from build123d import *

# Parameters (mm, degrees)
F0_W     = 127
F0_H     = 127
F1_DEPTH = 2.54
F2_W     = 127
F2_H     = 127
F2_W_2   = 121.92
F2_H_2   = 121.92
F3_DEPTH = 7.62
F4_W     = 5.08
F4_H     = 6.35
F4_W_2   = 7.62
F5_DEPTH = 15.24
F6_R     = 1.27
F6_W     = 5.08
F6_H     = 2.54
F7_DEPTH = 6.35


# Not quite as in the source:
# - a pattern or mirror of a feature is missing from the dataset's text; its kind, count and spacing are read off the source's solid


with BuildPart() as f1:
    # F0 (on Top) → F1 (new body)
    with BuildSketch(Plane.XY):
        Rectangle(F0_W, F0_H)
    extrude(amount=F1_DEPTH)

    # F2 (on face) → F3 (join)
    with BuildSketch(Plane.XY.offset(2.54)):
        Rectangle(F2_W, F2_H)
        Rectangle(F2_W_2, F2_H_2, mode=Mode.SUBTRACT)
    extrude(amount=F3_DEPTH)

    # F4 (on face) → F5 (join)
    with BuildSketch(Plane.XY.offset(2.54)):
        with Locations((-45.72, -41.275)):
            Rectangle(F4_W, F4_H)
        with Locations((45.72, -41.275)):
            Rectangle(F4_W_2, F4_H)
    f5 = extrude(amount=F5_DEPTH)

    # F5_copies: F5 across plane
    add(f5.mirror(Plane.ZX))

    # F6 (on face) → F7 (cut)
    with BuildSketch(Plane.XZ.offset(44.45)):
        with Locations((-45.72, 15.748)):
            Circle(F6_R)
        with Locations((45.72, 15.748)):
            Rectangle(F6_W, F6_H)
        with BuildLine():
            Line((-43.18, 17.78), (-45.72, 17.78))
            ThreePointArc((-45.72, 17.78), (-44.2831590206, 17.1848409794), (-43.688, 15.748))
            Line((-43.688, 15.748), (-43.18, 15.748))
            Line((-43.18, 15.748), (-43.18, 17.78))
        make_face()
        with BuildLine():
            ThreePointArc((-47.752, 15.748), (-47.1568409794, 17.1848409794), (-45.72, 17.78))
            Line((-45.72, 17.78), (-48.26, 17.78))
            Line((-48.26, 17.78), (-48.26, 15.748))
            Line((-48.26, 15.748), (-47.752, 15.748))
        make_face()
        with BuildLine():
            Line((49.7070066631, 17.7892204374), (45.72, 17.7892204374))
            ThreePointArc((45.72, 17.7892204374), (47.5717330447, 17.5942784861), (49.3422755435, 17.018))
            Line((49.3422755435, 17.018), (49.7070066631, 17.018))
            Line((49.7070066631, 17.018), (49.7070066631, 17.7892204374))
        make_face()
        with BuildLine():
            ThreePointArc((42.0977244565, 17.018), (43.8682669553, 17.5942784861), (45.72, 17.7892204374))
            Line((45.72, 17.7892204374), (41.827224195, 17.7892204374))
            Line((41.827224195, 17.7892204374), (41.827224195, 17.018))
            Line((41.827224195, 17.018), (42.0977244565, 17.018))
        make_face()
    f7 = extrude(amount=-F7_DEPTH, mode=Mode.SUBTRACT)

    # F7_copies: F7 across plane
    add(f7.mirror(Plane.ZX), mode=Mode.SUBTRACT)


solid = f1.part
Check sheet for the modelled part. Datum: model origin and axes. Units: mm. A direction names the side the tool comes from. Give positions to 0.01 mm unless a question says otherwise; leave off trailing zeros. Order: outer loops, then holes, each group sorted by start corner. A loop starts at its lowest first (then second) coordinate and runs counter-clockwise, first axis right, second up. Notation, with made-up numbers: M -22.5,72.5 L 26.5,72.5 A14 cw 26.5,86.5 Z; hole C -20.75,25.5 d3. An arc over 180 degrees is marked long. Answer as CSV lines item,"result". Start each with the question number.
Item 1: Cross-section at B-B on y = 51. Enter the section's corners in (x, z).
Item 2: Mould release check, pull along X, two halves, no side actions. Record for faces 1 (the face through (63.5, -1, 5)), 2 (the face through (-1, 63.5, 5)), 3 (the face through (-48.26, -41, 9)): +X half, -X half, draft (parallel to the pull), parting line (faces both ways), or undercut.
Item 3: Thickness scan on line 1 (X direction, y = -41.5, z = 9.5); line 2 (Y direction, x = -16.5, z = 5); line 3 (Z direction, x = -45.72, y = 39.5). Record the ranges inside material, lowest first. Write a range as [from, to].
Item 4: Cross-section at A-A on z = 6.5. Enter the section's corners in (x, y).
Item 5: Gauge pin test, flat ends, axial feed: P1, Ø4, axis at x = 45.5, y = -46.5, coming from the +Z side; P2, Ø0.8, axis at y = 40, z = 16, coming from the +X side; P3, Ø8, axis at y = 42.5, z = 14.5, coming from the -X side. Record the tip position at first contact, or that the pin passes through.
Item 6: Tool access check on faces 4 (the face through (46, -41, 14.478)), 5 (the face through (60.96, -1, 6)). Record the directions out of +Z, -Z, +X, -X, +Y, -Y that give a thin tool (end or side, any length) a straight path to the whole face; none if there is none.
Established:
1,outline,"M -63.5,0 L 63.5,0 L 63.5,10.16 L 60.96,10.16 L 60.96,2.54 L -60.96,2.54 L -60.96,10.16 L -63.5,10.16 Z"
2,face 1,"+X half"
2,face 2,"draft"
2,face 3,"undercut"
3,line 1,"x = [-63.5, -60.96], [-48.26, -43.18], [41.91, 49.53], [60.96, 63.5]"
3,line 2,"y = [-63.5, -60.96], [60.96, 63.5]"
3,line 3,"z = [0, 14.48], [17.02, 17.78]"
4,outline,"M -63.5,-63.5 L 63.5,-63.5 L 63.5,63.5 L -63.5,63.5 Z; M -48.26,-44.45 L -43.18,-44.45 L -43.18,-38.1 L -48.26,-38.1 Z; M -48.26,38.1 L -43.18,38.1 L -43.18,44.45 L -48.26,44.45 Z; M 41.91,-44.45 L 49.53,-44.45 L 49.53,-38.1 L 41.91,-38.1 Z; M 41.91,38.1 L 49.53,38.1 L 49.53,44.45 L 41.91,44.45 Z; hole M -60.96,-60.96 L 60.96,-60.96 L 60.96,60.96 L -60.96,60.96 Z"
5,P1,"stops at z = 2.54"
5,P2,"stops at x = 49.53"
5,P3,"stops at x = -48.26"
6,face 4,"+Y, -Y"
6,face 5,"+Z"
